Could you check a few things on this model? Use its own coordinates, in mm. Give positions to 0.01 mm unless a question says otherwise; leave off trailing zeros. Loops run counter-clockwise (first coordinate to the right, second up) from the corner with the lowest first, then second, coordinate; pieces in that order, holes last. Notation, with made-up numbers: (68.5, 27.25) - (106.5, 27.25) arc R34 cw to (106.5, 64.25) - close; hole circle Ø8 at (-12, 84.5). An arc over 180 degrees is marked (long way). Write each question's results on one line, items separated by ' | '. Start each with the question number.
(1) I need wall thicknesses on line 1 (Z direction, x = 0, y = -30); line 2 (X direction, y = -32, z = -2.5); line 3 (X direction, y = -38, z = -2). Which ranges of each line are inside material? Lowest first, please.
(2) For pin 1 (3 mm diameter, centred on x = 34.5, z = 18.5, fed in from -Y); pin 2 (10 mm diameter, centred on x = -13.5, z = -2, fed in from -Y); pin 3 (8 mm diameter, centred on x = 19, y = -15.5, fed in from +Z); pin 4 (1 mm diameter, centred on x = 10.5, y = -12.5, fed in from +Z), each with a flat end and sliding along its axis, tell me the tip position at first contact or that it passes through.
(3) Suppose I cut it at A-A (y = -9). Please give me the cut outline in (x, z) (3 decimals), and give its area (3 significant figures).
(4) Suppose I cut it at B-B (y = -38). Please give me the cut outline in (x, z), and give its area (3 significant figures).
(5) If we mould it in two halves opening along X, with no side actions, what happens to faces 1 (the face through (8.985, -21.914, 2.829)), 2 (the face through (36.935, -12.522, -17.064)), 3 (the face through (13, 0, 0))? For each: released by +X, released by -X, zero draft, split by the parting line, or undercut.
(6) Suppose I cut it at C-C (x = 40.5). Please give me the cut outline in (y, z).
from build123d import *

# Parameters (mm, degrees)
F0_R     = 9.419676
F0_R_2   = 6.35
F1_DEPTH = 25.4
F2_DEPTH = 50.8
F3_R     = 6.35
F4_SIZE  = 6.35
F5_SIZE  = 1.27


with BuildPart() as f1:
    # F0 (on Front) → F1 (new body)
    with BuildSketch(Plane.XZ):
        with BuildLine():
            ThreePointArc((6.072938, -24.663321), (19.992657, -15.666962), (25.4, 0))
            ThreePointArc((25.4, 0), (19.992657, 15.666962), (6.072938, 24.663321))
            ThreePointArc((6.072938, 24.663321), (-25.4, 0), (6.072938, -24.663321))
        make_face()
        Circle(F0_R, mode=Mode.SUBTRACT)
        with BuildLine():
            ThreePointArc((6.072938, 24.663321), (19.992657, 15.666962), (25.4, 0))
            ThreePointArc((25.4, 0), (19.992657, -15.666962), (6.072938, -24.663321))
            Line((6.072938, -24.663321), (68.674372, -9.248746))
            ThreePointArc((68.674372, -9.248746), (56.87202, 0), (68.674372, 9.248746))
            Line((68.674372, 9.248746), (6.072938, 24.663321))
        make_face()
        with BuildLine():
            ThreePointArc((75.92202, 0), (73.894266, 5.875111), (68.674372, 9.248746))
            ThreePointArc((68.674372, 9.248746), (56.87202, 0), (68.674372, -9.248746))
            ThreePointArc((68.674372, -9.248746), (73.894266, -5.875111), (75.92202, 0))
        make_face()
        with Locations((66.39702, 0)):
            Circle(F0_R_2, mode=Mode.SUBTRACT)
    extrude(amount=F1_DEPTH)

    # F0 (on Front) → F2 (join)
    with BuildSketch(Plane.XZ):
        with BuildLine():
            ThreePointArc((6.072938, -24.663321), (19.992657, -15.666962), (25.4, 0))
            ThreePointArc((25.4, 0), (19.992657, 15.666962), (6.072938, 24.663321))
            ThreePointArc((6.072938, 24.663321), (-25.4, 0), (6.072938, -24.663321))
        make_face()
        Circle(F0_R, mode=Mode.SUBTRACT)
    extrude(amount=F2_DEPTH)

    # F3
    f3_edges = [f1.edges().sort_by_distance(p)[0] for p in [
        (-6.072938, -50.8, 24.663321),
    ]]
    fillet(f3_edges, radius=F3_R)

    # F4
    f4_edges = [f1.edges().sort_by_distance(p)[0] for p in [
        (-9.419676, -50.8, 0),
    ]]
    chamfer(f4_edges, length=F4_SIZE)

    # F5
    f5_edges = [f1.edges().sort_by_distance(p)[0] for p in [
        (60.04702, -25.4, 0),
    ]]
    chamfer(f5_edges, length=F5_SIZE)


solid = f1.part
Output values:
1) line 1: -25.4 to -9.42, 9.42 to 25.4 | line 2: -25.28 to -9.08, 9.08 to 25.28 | line 3: -25.32 to -9.2, 9.2 to 25.32
2) pin 1: y = -25.4 | pin 2: y = -50.8 | pin 3: z = 22.47 | pin 4: z = 23.7
3) outline: (6.073, -24.663) - (68.674, -9.249) arc R9.525 ccw to (68.674, 9.249) - (6.073, 24.663) arc R25.4 ccw (long way) to start; hole circle Ø18.839 at (0, 0); hole circle Ø12.7 at (66.397, 0) | area: 3,140 mm2
4) outline: (6.07, -24.66) arc R25.4 ccw to (25.4, 0) arc R25.4 ccw to (6.07, 24.66) arc R25.4 ccw (long way) to start; hole circle Ø18.84 at (0, 0) | area: 1,750 mm2
5) face 1: undercut | face 2: released by +X | face 3: zero draft
6) outline: (-25.4, -16.19) - (0, -16.19) - (0, 16.19) - (-25.4, 16.19) - close
